```python
from build123d import *

# Parameters (mm, degrees)
F0_W     = 66.3625448942
F0_H     = 52.2382929921
F1_DEPTH = 25
F0_R     = 26.537616526


with BuildPart() as f1:
    # F0 (on Front) → F1 (new body)
    with BuildSketch(Plane.XZ):
        with Locations((-103.3144816756, 26.1191464961)):
            Rectangle(F0_W, F0_H)
    extrude(amount=F1_DEPTH)


with BuildPart() as f1b:
    # F0 (on Front) → F1, piece 2 (new body)
    with BuildSketch(Plane.XZ):
        with Locations((45.0334623456, 64.3185600638)):
            Circle(F0_R)
    extrude(amount=F1_DEPTH)


solid = f1b.part
```
CAD build for the part. Positions are in the model's coordinates, mm. Round coordinates to 2 decimals unless told otherwise and drop trailing zeros. Write each loop counter-clockwise with the first axis right and the second up, starting at its lowest first coordinate (ties: lowest second). Pieces come first, ordered by that corner, then holes. Notation, with made-up numbers: (-22.5, -33) - (36.5, -33) arc R17 cw to (36.5, -20) - close; hole circle Ø11 at (31.25, -26). An arc over 180 degrees is marked (long way). Return JSON: item names as keys, results as strings. Group by question number.
Item 1: Band-saw the part on A-A on z = 59. List the corners of the cut face in (x, y), plus the area to 3 significant figures.
Item 2: Band-saw the part on B-B on y = -21.25. List the corners of the cut face in (x, z), plus the area to 3 significant figures.
Item 3: Probe probe 1 along X at (y, z) = (-7.25, 80.5); probe 2 along X at (y, z) = (-6.25, 71); probe 3 along Z at (x, y) = (65, -2.5). List the from-to ranges inside material, lowest first.
Item 4: Flat gauge pins, fed straight in: pin 1 Ø5 at (y, z) = (-19.5, 61.5) entering from -X; pin 2 Ø8 at (y, z) = (-18, 53.5) entering from -X; pin 3 Ø4 at (x, y) = (27.5, -11) entering from +Z (3 decimals). Where does each tip first touch, or does it go through?
Item 5: Band-saw the part on C-C on x = 26.5. List the corners of the cut face in (y, z), plus the area to 3 significant figures.
Resolved:
{
 "1": {"outline": "(19.03, -25) - (71.03, -25) - (71.03, 0) - (19.03, 0) - close", "area": "1,300 mm²"},
 "2": {"outline": "circle Ø53.08 at (45.03, 64.32)", "area": "2,210 mm²"},
 "3": {"probe 1": "x = 24 to 66.07", "probe 2": "x = 19.35 to 70.72", "probe 3": "z = 46.84 to 81.8"},
 "4": {"pin 1": "stops at x = 18.5", "pin 2": "stops at x = 19.39", "pin 3": "stops at z = 85.835"},
 "5": {"outline": "(-25, 45.32) - (0, 45.32) - (0, 83.31) - (-25, 83.31) - close", "area": "950 mm²"}
}
